Source: three-view drawing plus pictorial views. Frame: mm from the lowest corner of the part. A direction names the side the tool comes from. Give positions to 0.01 mm unless a question says otherwise; leave off trailing zeros. Order: outer loops, then holes, each group sorted by start corner. A loop starts at its lowest first (then second) coordinate and runs counter-clockwise, first axis right, second up.
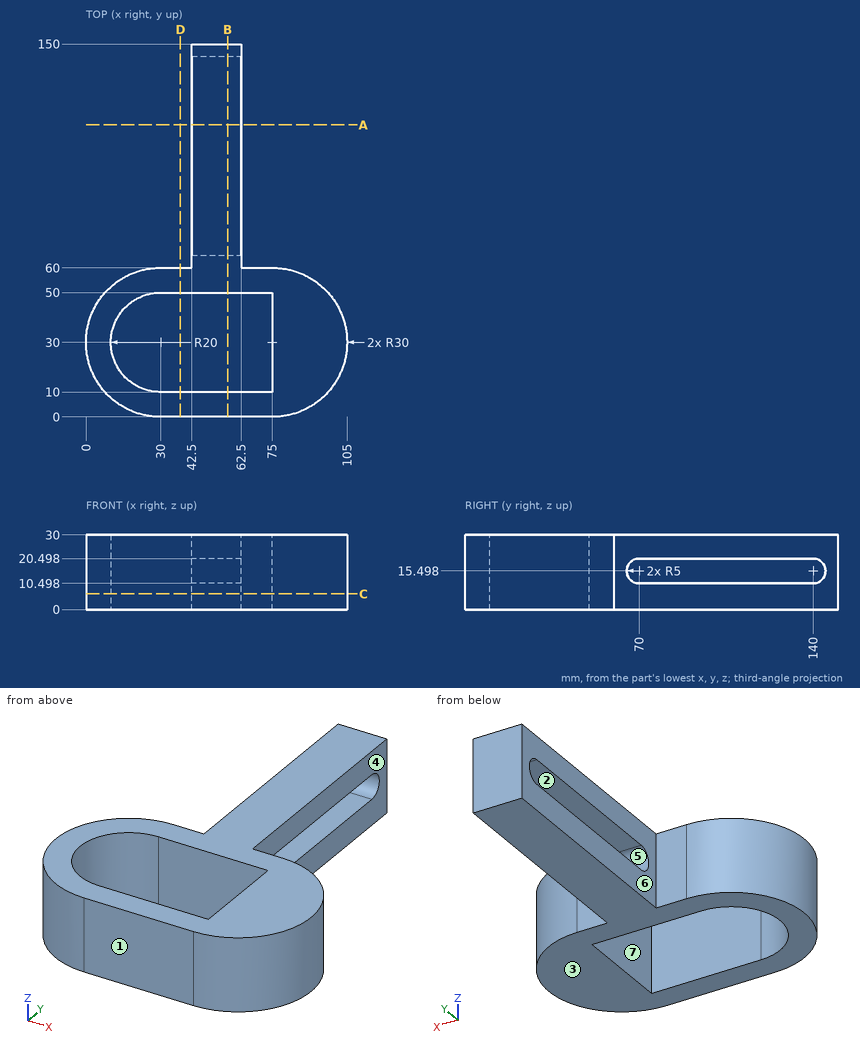
1) Ray query, L1, parallel to Y at x = 59.5, z = 26.5; L2, parallel to Y at x = 38.5, z = 15; L3, parallel to Y at x = 76, z = 26.75. Return the intervals inside material, ascending.
Checks:
L1: y = 0 to 10, 50 to 150
L2: y = 0 to 10, 50 to 60
L3: y = 0.02 to 59.98
2) Section query B-B on x = 57. Output: boundary loops of the cut face in (y, z).
Checks:
outline: (0, 0) - (10, 0) - (10, 30) - (0, 30) - close; (50, 0) - (150, 0) - (150, 30) - (50, 30) - close; hole (70, 10.5) - (140, 10.5) arc R5 ccw to (140, 20.5) - (70, 20.5) arc R5 ccw to start
3) Section query D-D on x = 38. Output: boundary loops of the cut face in (y, z).
Checks:
outline: (0, 0) - (10, 0) - (10, 30) - (0, 30) - close; (50, 0) - (60, 0) - (60, 30) - (50, 30) - close
4) Pull-direction query (Y, two-part tool) for the marked faces 1, 2 and 3; classes: +Y half, -Y half, draft (parallel to the pull), parting line (faces both ways), or undercut.
Checks:
face 1: -Y half
face 2: undercut
face 3: draft
5) First-contact query: pin 1 Ø8 at (y, z) = (23.5, 15) entering from -X; pin 2 Ø4 at (x, z) = (38.5, 10) entering from +Y; pin 3 Ø9 at (y, z) = (114, 17.5) entering from +X; pin 4 Ø9 at (y, z) = (106.5, 15.5) entering from -X. Flat tips, straight axial feed; report the tip coordinate or a pass-through.
Checks:
pin 1: stops at x = 0.1
pin 2: stops at y = 60
pin 3: stops at x = 62.5
pin 4: passes through
6) Section query A-A on y = 117.5. Output: boundary loops of the cut face in (x, z).
Checks:
outline: (42.5, 0) - (62.5, 0) - (62.5, 10.5) - (42.5, 10.5) - close; (42.5, 20.5) - (62.5, 20.5) - (62.5, 30) - (42.5, 30) - close
7) Reachability of the marked faces 4, 5, 6 and 7 from +Z, -Z, +X, -X, +Y, -Y: full face, straight path, thin tool, end or side. Return the list, or none.
Checks:
face 4: +Z, -Z, +X, +Y
face 5: +X, -X
face 6: +Z, -Z, -X, +Y
face 7: +Z, -Z
8) Section query C-C on z = 6.25. Output: boundary loops of the cut face in (x, y).
Checks:
outline: (30, 0) - (75, 0) arc R30 ccw to (75, 60) - (62.5, 60) - (62.5, 150) - (42.5, 150) - (42.5, 60) - (30, 60) arc R30 ccw to start; hole (30, 10) - (75, 10) - (75, 50) - (30, 50) arc R20 ccw to start
